Design review of the part shown in the three views and the two pictorial views. Dimensions are in mm from the part's minimum x, y and z. Give positions to 0.01 mm unless a question says otherwise; leave off trailing zeros. Loops run counter-clockwise (first coordinate to the right, second up) from the corner with the lowest first, then second, coordinate; pieces in that order, holes last. Notation, with made-up numbers: (0.25, 28.25) - (12.25, 28.25) arc R20 cw to (12.25, 36.25) - close; hole circle Ø11 at (71.5, 41.25). An arc over 180 degrees is marked (long way). Answer as a JSON object with one key per item and string values.
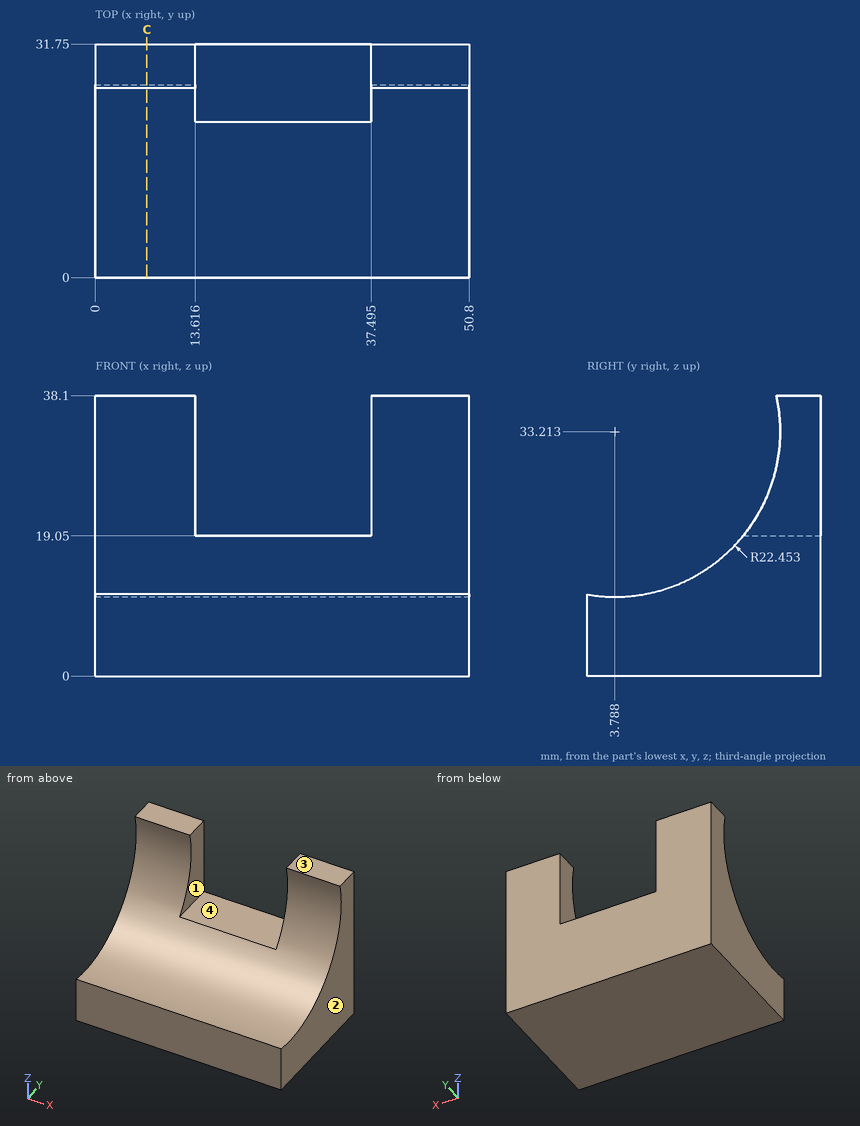
Q1. To check wall thickness, follow probe 1 along Z at (x, y) = (19, 23); probe 2 along Y at (x, z) = (46.5, 33); probe 3 along Z at (x, y) = (9, 18.5). State the ranges of each line that lie inside material, in increasing order. Write a range as [from, to].
Results:
{"probe 1": "z = [0, 19.05]", "probe 2": "y = [26.24, 31.75]", "probe 3": "z = [0, 16.25]"}
Q2. Consider section C-C, the plane x = 7. State the section outline as (y, z) points, plus the area to 3 significant figures.
Results:
{"outline": "(0, 0) - (31.75, 0) - (31.75, 38.1) - (25.7, 38.1) arc R22.45 cw to (0, 11.08) - close", "area": "602 mm^2"}
Q3. The part is to be moulded in two halves that separate along X. For the marked faces 1, 2, 3 and 4, say which applies: +X half, -X half, draft (parallel to the pull), parting line (faces both ways), or undercut.
Results:
{"face 1": "undercut", "face 2": "+X half", "face 3": "draft", "face 4": "undercut"}
Q4. Clearance check with flat-ended pins moving along their axes: pin 1 Ø2 at (x, z) = (36, 25.5) entering from -Y; pin 2 Ø3 at (y, z) = (24.5, 26.5) entering from -X; pin 3 Ø3 at (x, y) = (24.5, 24.5) entering from +Z; pin 4 Ø8 at (x, z) = (33.5, 18.5) entering from -Y (1 decimal). State where each tip first meets the part, or that it passes through.
Results:
{"pin 1": "passes through", "pin 2": "stops at x = 0", "pin 3": "stops at z = 19.05", "pin 4": "stops at y = 16.2"}
